Could you check a few things on this model? Use its own coordinates, in mm. Face numbers are marked on the shaded views. Round coordinates to 2 decimals unless told otherwise and drop trailing zeros. Loops run counter-clockwise (first coordinate to the right, second up) from the corner with the lowest first, then second, coordinate; pieces in that order, holes last. Notation, with made-up numbers: (33, 85.25) -> (89, 85.25) arc R19 ccw to (89, 107.25) -> close; hole circle Ø5 at (89.25, 46). An arc over 180 degrees is marked (long way). Write each question's results on one line, items separated by ' | '.
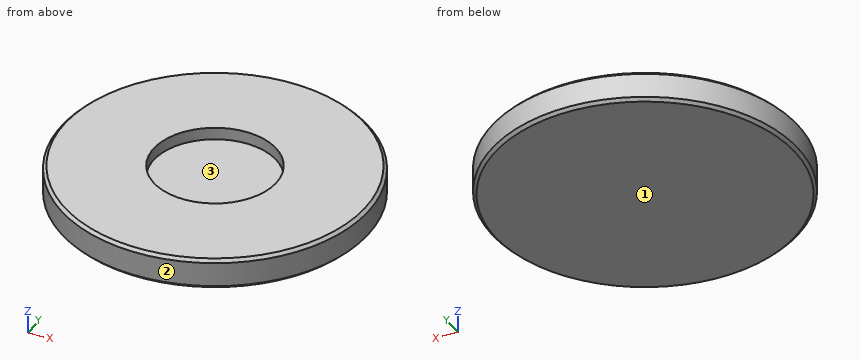
from build123d import *

# Parameters (mm, degrees)
F0_R     = 50
F1_DEPTH = 10
F2_R     = 20
F3_DEPTH = 4
F4_SIZE  = 1


with BuildPart() as f1:
    # F0 (on Top) → F1 (new body)
    with BuildSketch(Plane.XY):
        Circle(F0_R)
    extrude(amount=F1_DEPTH)

    # F2 (on face) → F3 (cut)
    with BuildSketch(Plane.XY.offset(10)):
        Circle(F2_R)
    extrude(amount=-F3_DEPTH, mode=Mode.SUBTRACT)

    # F4
    f4_edges = [f1.edges().sort_by_distance(p)[0] for p in [
        (-50, 0, 10),
        (-50, 0, 0),
    ]]
    chamfer(f4_edges, length=F4_SIZE)


solid = f1.part
1) I want a section at A-A, the plane y = 0. Write out the boundary of the cut face in (x, z), plus the area to 3 significant figures.
Model answer:
outline: (-50, 1) -> (-49, 0) -> (49, 0) -> (50, 1) -> (50, 9) -> (49, 10) -> (20, 10) -> (20, 6) -> (-20, 6) -> (-20, 10) -> (-49, 10) -> (-50, 9) -> close | area: 838 mm2
2) I need wall thicknesses on line 1 (Y direction, x = 0, z = 7.4); line 2 (Z direction, x = -8.5, y = 4.5); line 3 (X direction, y = 17.5, z = 7.5). Which ranges of each line are inside material? Lowest first, please.
Model answer:
line 1: y = -50 to -20, 20 to 50 | line 2: z = 0 to 6 | line 3: x = -46.84 to -9.68, 9.68 to 46.84
3) If we mould it in two halves opening along Y, with no side actions, what happens to the marked faces 1, 2 and 3? For each: released by +Y, released by -Y, zero draft, split by the parting line, or undercut.
Model answer:
face 1: zero draft | face 2: split by the parting line | face 3: undercut
4) I'm going to push flat-ended pins straight in: pin 1 (6 mm diameter, centred on y = 8, z = 2, fed in from -X); pin 2 (5 mm diameter, centred on y = 25.5, z = 2, fed in from -X); pin 3 (1.5 mm diameter, centred on y = 19.5, z = 3.5, fed in from -X). Where does each tip first touch, or does it pass through?
Model answer:
pin 1: stops at x = -49.75 | pin 2: stops at x = -44.4 | pin 3: stops at x = -46.35
